Can you work these out from the drawing? Everything is in mm from the part's minimum corner. A direction names the side the tool comes from. Give positions to 0.01 mm unless a question says otherwise; leave off trailing zeros. Order: outer loops, then holes, each group sorted by start corner. A loop starts at its lowest first (then second) coordinate and runs counter-clockwise, first axis right, second up. Notation, with made-up numbers: M 11,10.25 L 62,10.25 A22 ccw 62,33.25 Z; hole C 25.25,4 d11. An arc over 180 degrees is marked long. Answer as a JSON object with one key per item and string values.
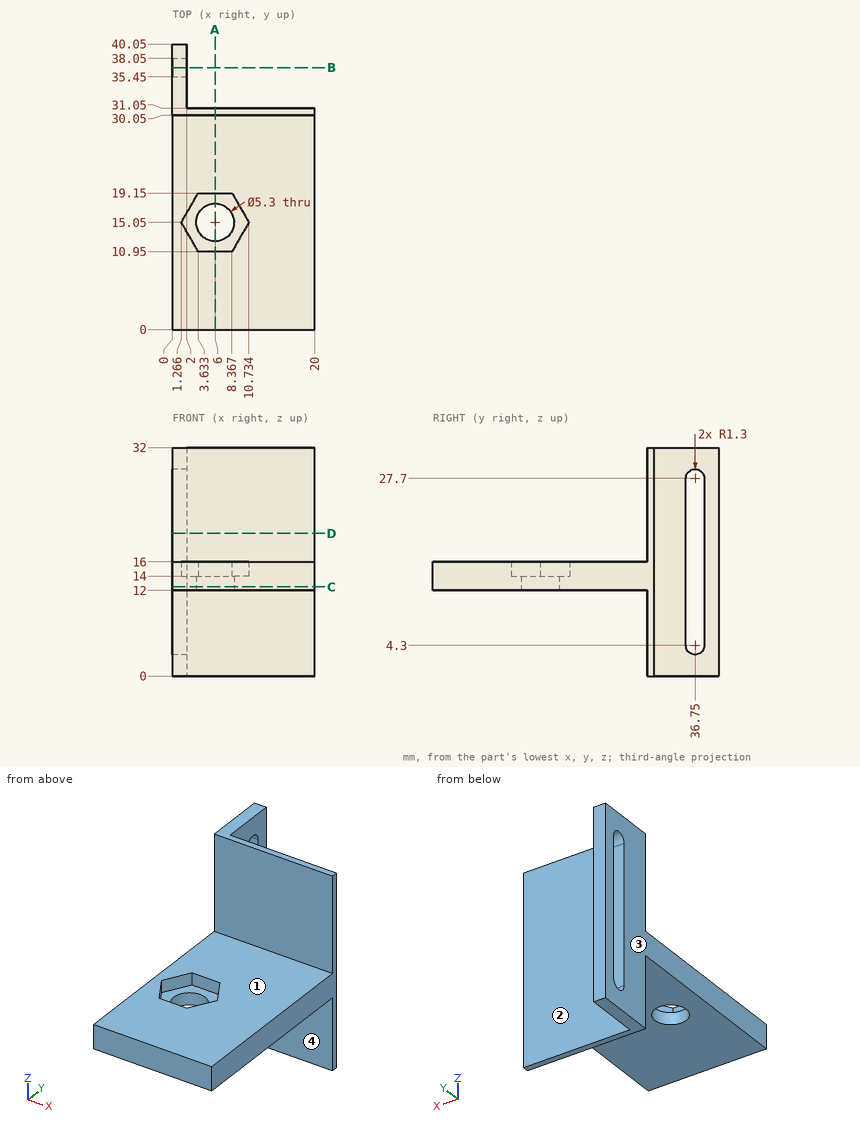
1) I want a section at B-B on y = 36.75. Write out the boundary of the cut face in (x, z).
Results found:
{"outline": "M 0,0 L 2,0 L 2,3 L 0,3 Z; M 0,29 L 2,29 L 2,32 L 0,32 Z"}
2) I need wall thicknesses on L1, parallel to X at y = 15.05, z = 13.45; L2, parallel to Y at x = 6, z = 12.7; L3, parallel to X at y = 38.5, z = 31. Which ranges of each line are inside material? Lowest first, please.
Results found:
{"L1": "x = 0 to 3.35, 8.65 to 20", "L2": "y = 0 to 12.4, 17.7 to 31.05", "L3": "x = 0 to 2"}
3) For the marked faces 1, 2, 3 and 4, which set-ups out of +Z, -Z, +X, -X, +Y, -Y let a thin tool reach every point of the face, with its end or its side?
Results found:
{"face 1": "+Z, +X, -X, -Y", "face 2": "+Z, -Z, +X, +Y", "face 3": "+Z, -Z, -X, +Y, -Y", "face 4": "-Z, +X, -X, -Y"}
4) I want a section at A-A on x = 6. Write out the boundary of the cut face in (y, z).
Results found:
{"outline": "M 0,12 L 12.4,12 L 12.4,14 L 10.95,14 L 10.95,16 L 0,16 Z; M 17.7,12 L 30.05,12 L 30.05,0 L 31.05,0 L 31.05,32 L 30.05,32 L 30.05,16 L 19.15,16 L 19.15,14 L 17.7,14 Z"}
5) I want a section at D-D on z = 20. Write out the boundary of the cut face in (x, y), and give its area (3 significant figures).
Results found:
{"outline": "M 0,30.05 L 20,30.05 L 20,31.05 L 2,31.05 L 2,35.45 L 0,35.45 Z; M 0,38.05 L 2,38.05 L 2,40.05 L 0,40.05 Z", "area": "32.8 mm²"}
6) I want a section at C-C on z = 12.5. Write out the boundary of the cut face in (x, y), and give its area (3 significant figures).
Results found:
{"outline": "M 0,0 L 20,0 L 20,31.05 L 2,31.05 L 2,35.45 L 0,35.45 Z; M 0,38.05 L 2,38.05 L 2,40.05 L 0,40.05 Z; hole C 6,15.05 d5.3", "area": "612 mm²"}
7) I'm going to push flat-ended pins straight in: pin 1 Ø0.6 at (x, z) = (6.5, 15) entering from +Y; pin 2 Ø10 at (x, y) = (14, 19) entering from -Z; pin 3 Ø6 at (x, z) = (7.5, 6.5) entering from -Y; pin 4 Ø2.5 at (x, y) = (6, 15) entering from +Z. Where does each tip first touch, or does it pass through?
Results found:
{"pin 1": "stops at y = 31.05", "pin 2": "stops at z = 12", "pin 3": "stops at y = 30.05", "pin 4": "passes through"}
